Can you work these out from the model? Positions are in its coordinate system, mm. Round coordinates to 2 decimals unless told otherwise and drop trailing zeros. Order: outer loops, then holes, each group sorted by start corner. A loop starts at its lowest first (then second) coordinate and runs counter-clockwise, first axis right, second up. Notation, with made-up numbers: (37.25, 3.25) - (83.25, 3.25) arc R11 ccw to (83.25, 10.25) - close; hole circle Ø9 at (48, 7.5). An arc over 180 degrees is marked (long way). Write item = value, one per line.
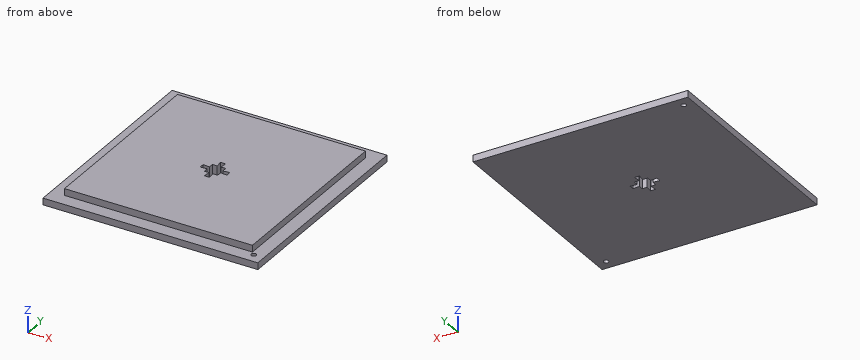
from build123d import *

# Parameters (mm, degrees)
F0_W      = 81.28
F0_H      = 81.28
F1_DEPTH  = 38.1
F2_W      = 81.28
F2_H      = 81.28
F2_W_2    = 71.12
F2_H_2    = 71.12
F3_DEPTH  = 35.56
F4_W      = 76.2
F4_H      = 76.2
F5_DEPTH  = 33.02
F7_DEPTH  = 25.4
F8_R      = 0.9525
F9_DEPTH  = 25.4
F10_R     = 0.9525
F11_DEPTH = 25.4


with BuildPart() as f1:
    # F0 (on Top) → F1 (new body)
    with BuildSketch(Plane.XY):
        Rectangle(F0_W, F0_H)
    extrude(amount=F1_DEPTH)

    # F2 (on face) → F3 (cut)
    with BuildSketch(Plane.XY.offset(38.1)):
        Rectangle(F2_W, F2_H)
        Rectangle(F2_W_2, F2_H_2, mode=Mode.SUBTRACT)
    extrude(amount=-F3_DEPTH, mode=Mode.SUBTRACT)

    # F4 (on face) → F5 (cut)
    with BuildSketch(Plane.XY.offset(38.1)):
        Rectangle(F4_W, F4_H)
    extrude(amount=-F5_DEPTH, mode=Mode.SUBTRACT)

    # F6 (on face) → F7 (cut)
    with BuildSketch(Plane.XY.offset(5.08)):
        Polygon((-0.9525, -5.067268), (0.9525, -5.067268), (0.6985, -2.54), (2.54, -2.54), (2.54, -0.6985), (5.067268, -0.9525), (5.067268, 0.9525), (2.54, 0.6985), (2.54, 2.54), (0.6985, 2.54), (0.9525, 5.067268), (-0.9525, 5.067268), (-0.6985, 2.54), (-2.54, 2.54), (-2.54, 0.6985), (-5.067268, 0.9525), (-5.067268, -0.9525), (-2.54, -0.6985), (-2.54, -2.54), (-0.6985, -2.54), align=None)
    extrude(amount=-F7_DEPTH, mode=Mode.SUBTRACT)

    # F8 (on face) → F9 (cut)
    with BuildSketch(Plane.XY.offset(2.54)):
        with Locations((-36.83, 36.83)):
            Circle(F8_R)
    extrude(amount=-F9_DEPTH, mode=Mode.SUBTRACT)

    # F10 (on face) → F11 (cut)
    with BuildSketch(Plane.XY.offset(2.54)):
        with Locations((36.83, -36.83)):
            Circle(F10_R)
    extrude(amount=-F11_DEPTH, mode=Mode.SUBTRACT)


solid = f1.part
(1) If we section it at C-C (y = -36.83): Write out the boundary of the cut face in (x, z).
Computed:
outline = (-40.64, 0) - (35.88, 0) - (35.88, 2.54) - (-40.64, 2.54) - close; (37.78, 0) - (40.64, 0) - (40.64, 2.54) - (37.78, 2.54) - close
(2) Will these pins go through, and if not, where does the flat tip stop? P1, Ø0.8, axis at y = -7, z = 4, coming from the +X side; P2, Ø1.5, axis at x = 0, z = 3, coming from the -Y side; P3, Ø0.6, axis at x = -1.5, z = 3.5, coming from the -Y side; P4, Ø1.5, axis at x = 36.83, y = -36.83, coming from the +Z side.
Computed:
P1 = 35.56
P2 = -40.64
P3 = -35.56
P4 = through
(3) If we section it at B-B (x = 36.83): Write out the boundary of the cut face in (y, z), plus the area to 3 significant figures.
Computed:
outline = (-40.64, 0) - (-37.78, 0) - (-37.78, 2.54) - (-40.64, 2.54) - close; (-35.88, 0) - (40.64, 0) - (40.64, 2.54) - (-35.88, 2.54) - close
area = 202 mm^2
(4) If we section it at A-A (z = 3.6): Write out the boundary of the cut face in (x, y).
Computed:
outline = (-35.56, -35.56) - (35.56, -35.56) - (35.56, 35.56) - (-35.56, 35.56) - close; hole (-5.07, -0.95) - (-2.54, -0.7) - (-2.54, -2.54) - (-0.7, -2.54) - (-0.95, -5.07) - (0.95, -5.07) - (0.7, -2.54) - (2.54, -2.54) - (2.54, -0.7) - (5.07, -0.95) - (5.07, 0.95) - (2.54, 0.7) - (2.54, 2.54) - (0.7, 2.54) - (0.95, 5.07) - (-0.95, 5.07) - (-0.7, 2.54) - (-2.54, 2.54) - (-2.54, 0.7) - (-5.07, 0.95) - close
(5) If we section it at D-D (x = 25): Write out the boundary of the cut face in (y, z), plus the area to 3 significant figures.
Computed:
outline = (-40.64, 0) - (40.64, 0) - (40.64, 2.54) - (35.56, 2.54) - (35.56, 5.08) - (-35.56, 5.08) - (-35.56, 2.54) - (-40.64, 2.54) - close
area = 387 mm^2
(6) If I drill on line 1 (Y direction, x = -36.83, z = 1.7); line 2 (Y direction, x = 36.83, z = 0.7), over which ranges is the centre line in solid material (lowest first)? Write a range as from..to.
Computed:
line_1 = -40.64..35.88, 37.78..40.64
line_2 = -40.64..-37.78, -35.88..40.64
